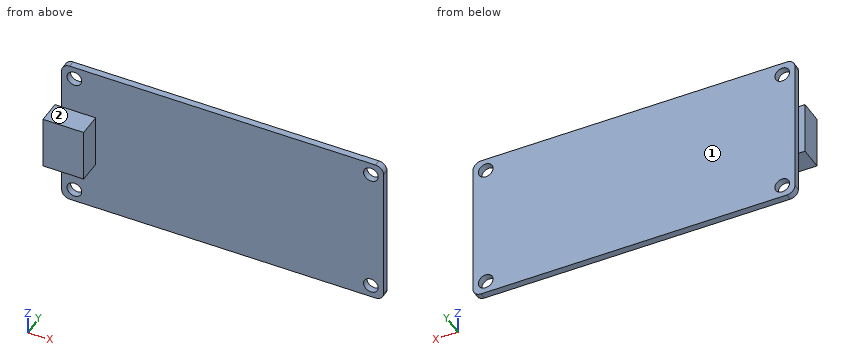
from build123d import *

# Parameters (mm, degrees)
SKETCH1_W               = 48.26
SKETCH1_H               = 22.86
BOSS_EXTRUDE1_DEPTH     = 1
SKETCH2_R               = 1.09982
CUT_EXTRUDE1_DEPTH      = 1
CUT_EXTRUDE1_DEPTH_BACK = 2
FILLET1_R               = 1.2065
SKETCH3_W               = 6.1
SKETCH3_H               = 8
BOSS_EXTRUDE2_DEPTH     = 3.5


with BuildPart() as part:
    # Sketch1 → Boss-Extrude1 (new body)
    with BuildSketch(Plane(origin=(0, 0, 0), x_dir=(1, 0, 0), z_dir=(0, 1, 0))):
        with Locations((24.13, 11.43)):
            Rectangle(SKETCH1_W, SKETCH1_H)
    extrude(amount=BOSS_EXTRUDE1_DEPTH)

    # Sketch2 → Cut-Extrude1 (cut, two sides)
    with BuildSketch(Plane(origin=(0, 1, 0), x_dir=(1, 0, 0), z_dir=(0, 1, 0))) as cut_extrude1_sk:
        with Locations((1.905, 20.955)):
            Circle(SKETCH2_R)
        with Locations((1.905, 1.905)):
            Circle(SKETCH2_R)
        with Locations((46.355, 1.905)):
            Circle(SKETCH2_R)
        with Locations((46.355, 20.955)):
            Circle(SKETCH2_R)
    extrude(amount=CUT_EXTRUDE1_DEPTH, mode=Mode.SUBTRACT)
    extrude(cut_extrude1_sk.sketch, amount=-CUT_EXTRUDE1_DEPTH_BACK, mode=Mode.SUBTRACT)

    # Fillet1
    fillet1_edges = [part.edges().sort_by_distance(p)[0] for p in [
        (0, 0.5, -22.86),
        (48.26, 0.5, -22.86),
        (48.26, 0.5, 0),
        (0, 0.5, 0),
    ]]
    fillet(fillet1_edges, radius=FILLET1_R)

    # Sketch3 → Boss-Extrude2 (add)
    with BuildSketch(Plane.XZ):
        with Locations((2.05, -11.43)):
            Rectangle(SKETCH3_W, SKETCH3_H)
    extrude(amount=BOSS_EXTRUDE2_DEPTH)


solid = part.part
Work out the finished part from the listing and answer in its coordinate system (mm). Face numbers are marked on the shaded views. A direction names the side the tool comes from. Round coordinates to 2 decimals unless told otherwise and drop trailing zeros. Order: outer loops, then holes, each group sorted by start corner. A loop starts at its lowest first (then second) coordinate and runs counter-clockwise, first axis right, second up. Notation, with made-up numbers: M -18,23.25 L 29,23.25 A25 ccw 29,62.25 Z; hole C -29.5,69.5 d8. An arc over 180 degrees is marked long. One line per item, written item: value.
Q1. Find section A-A on z = -2.5. Write down the section's boundary in (x, y).
Derived:
outline: M 0,0 L 0.98,0 L 0.98,1 L 0,1 Z; M 2.83,0 L 45.43,0 L 45.43,1 L 2.83,1 Z; M 47.28,0 L 48.26,0 L 48.26,1 L 47.28,1 Z
Q2. Flat-ended cylindrical pins translate along their axes: pin 1 (3.5 mm diameter, centred on x = 46.355, z = -20.955, fed in from +Y); pin 2 (10 mm diameter, centred on x = 25, z = -20, fed in from -Y); pin 3 (1.5 mm diameter, centred on y = -1, z = -14.5, fed in from +X); pin 4 (1.1 mm diameter, centred on y = 0.5, z = -16, fed in from -X). Find the tip coordinate at first contact, or state that the pin passes through.
Derived:
pin 1: y = 1
pin 2: y = 0
pin 3: x = 5.1
pin 4: x = 0
Q3. Find section B-B on z = -9. Write down the section's boundary in (x, y).
Derived:
outline: M -1,-3.5 L 5.1,-3.5 L 5.1,0 L 48.26,0 L 48.26,1 L 0,1 L 0,0 L -1,0 Z
Q4. Find section D-D on x = 23.5. Write down the section's boundary in (y, z).
Derived:
outline: M 0,-22.86 L 1,-22.86 L 1,0 L 0,0 Z
Q5. For the marked faces 1 and 2, determine the directions among +Z, -Z, +X, -X, +Y, -Y from which every point of the face is accessible in a straight line to the end or side of a thin tool.
Derived:
face 1: +Z, -Z, +X, -X, +Y
face 2: +Z, +X, -X, -Y
Q6. Straight lines are drawn through the part: line 1 (Z direction, x = 2.5, y = -1.4); line 2 (Y direction, x = 38, z = -8.5); line 3 (X direction, y = 0.45, z = -16.75). For each, find the intervals that lie inside material, in ascending order.
Derived:
line 1: -15.43 to -7.43
line 2: 0 to 1
line 3: 0 to 48.26
Q7. Find section C-C on y = -2.35. Write down the section's boundary in (x, z), then the cut area to 3 significant figures.
Derived:
outline: M -1,-15.43 L 5.1,-15.43 L 5.1,-7.43 L -1,-7.43 Z
area: 48.8 mm²
